Verification items for the finished model (mm, model axes). A direction names the side the tool comes from. Round coordinates to 2 decimals unless told otherwise and drop trailing zeros. Loops run counter-clockwise (first coordinate to the right, second up) from the corner with the lowest first, then second, coordinate; pieces in that order, holes last. Notation, with made-up numbers: (21.25, -19) - (36.25, -19) arc R24 ccw to (36.25, 13) - close; hole circle Ø11 at (3.5, 79). An arc over 180 degrees is marked (long way). Use a Markdown table: item, result. Add a question column.
```python
from build123d import *

# Parameters (mm, degrees)
SKETCH_W               = 110.32
SKETCH_H               = 165.5
PAD_DEPTH              = 6.4
SKETCH001_W            = 80.32
SKETCH001_H            = 135.5
POCKET_DEPTH           = 6.401
SKETCH002_R            = 5.025
POCKET001_DEPTH        = 1.645
LINEARPATTERN_COUNT    = 2
LINEARPATTERN_PITCH    = 40
LINEARPATTERN001_COUNT = 2
LINEARPATTERN001_PITCH = 40


with BuildPart() as part:
    # Sketch → Pad (new body)
    with BuildSketch(Plane.XY):
        Rectangle(SKETCH_W, SKETCH_H)
    extrude(amount=PAD_DEPTH)

    # Sketch001 → Pocket (cut, through all)
    with BuildSketch(Plane.XY.offset(6.4)):
        Rectangle(SKETCH001_W, SKETCH001_H)
    extrude(amount=-POCKET_DEPTH, mode=Mode.SUBTRACT)

    # Sketch002 → Pocket001 (cut)
    with BuildSketch(Plane.XY.offset(6.4)):
        with Locations((0, 75.25)):
            Circle(SKETCH002_R)
        with Locations((0, -75.25)):
            Circle(SKETCH002_R)
    pocket001 = extrude(amount=-POCKET001_DEPTH, mode=Mode.SUBTRACT)

    # LinearPattern: Pocket001 ×2
    with Locations(*[(i * LINEARPATTERN_PITCH, 0, 0) for i in range(1, LINEARPATTERN_COUNT)]):
        add(pocket001, mode=Mode.SUBTRACT)

    # LinearPattern001: Pocket001 ×2
    with Locations(*[(-i * LINEARPATTERN001_PITCH, 0, 0) for i in range(1, LINEARPATTERN001_COUNT)]):
        add(pocket001, mode=Mode.SUBTRACT)


solid = part.part
```
Q1. Section check A-A on x = 0. Record the cut outline in (y, z) (3 decimals).
Q2. Thickness scan on line 1 along Y through (x, z) = (0, 6) (3 decimals); line 2 along X through (y, z) = (-8.5, 3); line 3 along Y through (x, z) = (-32.5, 0.75). Record the ranges inside material, lowest first.
Q3. Release check for a two-part mould opening along X. For faces 4 (the face through (-1.089, 70.344, 5.589)), 5 (the face through (-1, 82.75, 3)), 6 (the face through (-55.16, -1, 3)) record: +X half, -X half, draft (parallel to the pull), parting line (faces both ways), or undercut.
Q4. Go/stop test with flat-tipped pins: pin 1 Ø11 at (x, y) = (0.5, 75.5) entering from +Z; pin 2 Ø3 at (x, y) = (39, 77) entering from +Z (3 decimals). Record where each tip stops, or that it passes through.
Q5. Section check D-D on y = 75.25. Record the cut outline in (x, z) (3 decimals), plus the area to 3 significant figures.
Q6. Section check C-C on y = -62. Record the cut outline in (x, z).
Q7. Section check B-B on z = 1.75. Record the cut outline in (x, y), plus the area to 3 significant figures.
Q8. Set-up check for faces 1 (the face through (-50, 1, 0)), 2 (the face through (40.16, -1, 3)), 3 (the face through (40, -75, 4.755)): record each of +Z, -Z, +X, -X, +Y, -Y from which the full face is reachable in a straight line by a thin tool's end or side.
Determined:
| question | item | result |
|---|---|---|
| 1 | outline | (-82.75, 0) - (-67.75, 0) - (-67.75, 6.4) - (-70.225, 6.4) - (-70.225, 4.755) - (-80.275, 4.755) - (-80.275, 6.4) - (-82.75, 6.4) - close; (67.75, 0) - (82.75, 0) - (82.75, 6.4) - (80.275, 6.4) - (80.275, 4.755) - (70.225, 4.755) - (70.225, 6.4) - (67.75, 6.4) - close |
| 2 | line 1 | y = -82.75 to -80.275, -70.225 to -67.75, 67.75 to 70.225, 80.275 to 82.75 |
| 2 | line 2 | x = -55.16 to -40.16, 40.16 to 55.16 |
| 2 | line 3 | y = -82.75 to -67.75, 67.75 to 82.75 |
| 3 | face 4 | undercut |
| 3 | face 5 | draft |
| 3 | face 6 | -X half |
| 4 | pin 1 | stops at z = 6.4 |
| 4 | pin 2 | stops at z = 4.755 |
| 5 | outline | (-55.16, 0) - (55.16, 0) - (55.16, 6.4) - (45.025, 6.4) - (45.025, 4.755) - (34.975, 4.755) - (34.975, 6.4) - (5.025, 6.4) - (5.025, 4.755) - (-5.025, 4.755) - (-5.025, 6.4) - (-34.975, 6.4) - (-34.975, 4.755) - (-45.025, 4.755) - (-45.025, 6.4) - (-55.16, 6.4) - close |
| 5 | area | 656 mm² |
| 6 | outline | (-55.16, 0) - (-40.16, 0) - (-40.16, 6.4) - (-55.16, 6.4) - close; (40.16, 0) - (55.16, 0) - (55.16, 6.4) - (40.16, 6.4) - close |
| 7 | outline | (-55.16, -82.75) - (55.16, -82.75) - (55.16, 82.75) - (-55.16, 82.75) - close; hole (-40.16, -67.75) - (40.16, -67.75) - (40.16, 67.75) - (-40.16, 67.75) - close |
| 7 | area | 7,370 mm² |
| 8 | face 1 | -Z, +X, -X, +Y, -Y |
| 8 | face 2 | +Z, -Z |
| 8 | face 3 | +Z |
